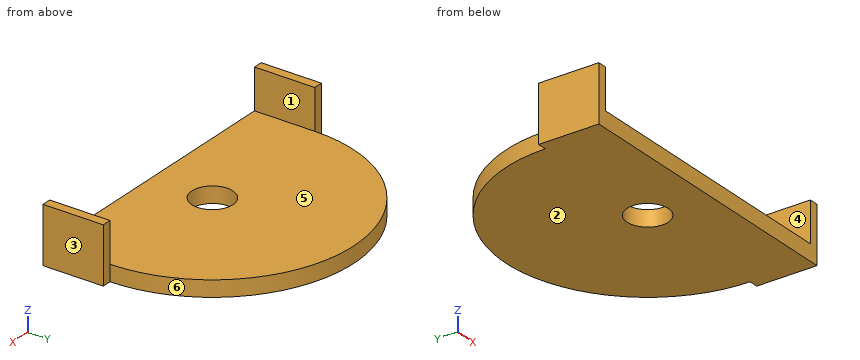
from build123d import *

# Parameters (mm, degrees)
F0_R     = 6.477
F1_DEPTH = 5.08
F2_W     = 2.921
F2_H     = 19.05
F3_DEPTH = 12.7


with BuildPart() as f1:
    # F0 (on Top) → F1 (new body)
    with BuildSketch(Plane.XY):
        with BuildLine():
            Line((47.625, 0), (44.704, 0))
            ThreePointArc((44.704, 0), (0, 44.704), (-44.704, 0))
            Line((-44.704, 0), (-47.625, 0))
            Line((-47.625, 0), (-47.625, -19.05))
            Line((-47.625, -19.05), (47.625, -19.05))
            Line((47.625, -19.05), (47.625, 0))
        make_face()
        Circle(F0_R, mode=Mode.SUBTRACT)
    extrude(amount=F1_DEPTH)

    # F2 (on face) → F3 (join)
    with BuildSketch(Plane.XY.offset(5.08)):
        with Locations((-46.1645, -9.525)):
            Rectangle(F2_W, F2_H)
        with Locations((46.1645, -9.525)):
            Rectangle(F2_W, F2_H)
    extrude(amount=F3_DEPTH)


solid = f1.part
Build history of the part. All positions in model axes, mm. Face numbers are marked on the shaded views. A direction names the side the tool comes from. Round coordinates to 2 decimals unless told otherwise and drop trailing zeros. Write each loop counter-clockwise with the first axis right and the second up, starting at its lowest first coordinate (ties: lowest second). Pieces come first, ordered by that corner, then holes. Notation, with made-up numbers: M 72,75.25 L 89,75.25 A21 ccw 89,83.25 Z; hole C 83.5,56.5 d10. An arc over 180 degrees is marked long. Answer in a Markdown table with one row per item.
1. Saw through at D-D (y = -12). List the corners of the cut face in (x, z) (3 decimals), and give its area (3 significant figures).
Geometry check:
| item | result |
|---|---|
| outline | M -47.625,0 L 47.625,0 L 47.625,17.78 L 44.704,17.78 L 44.704,5.08 L -44.704,5.08 L -44.704,17.78 L -47.625,17.78 Z |
| area | 558 mm2 |
2. Mould opens along X. For the marked faces 1, 2, 3 and 4 say: +X half, -X half, draft (parallel to the pull), parting line (faces both ways), or undercut.
Geometry check:
| item | result |
|---|---|
| face 1 | undercut |
| face 2 | draft |
| face 3 | +X half |
| face 4 | undercut |
3. Which spindle directions (+Z, -Z, +X, -X, +Y, -Y) get a long thin tool onto all of the face, cutting with end or side? Do the marked faces 5 and 6. Say none if no direction does.
Geometry check:
| item | result |
|---|---|
| face 5 | +Z, +Y, -Y |
| face 6 | +Z, -Z, +Y |
4. Flat gauge pins, fed straight in: P1, Ø3, axis at x = 46.5, z = 7.5, coming from the +Y side; P2, Ø4, axis at y = 6, z = 4.5, coming from the -X side; P3, Ø4, axis at x = 14, y = 19, coming from the +Z side; P4, Ø15, axis at x = 0, y = 0, coming from the -Z side. Where does each tip first touch, or does it go through?
Geometry check:
| item | result |
|---|---|
| P1 | y = 0 |
| P2 | x = -44.52 |
| P3 | z = 5.08 |
| P4 | z = 0 |
5. Probe L1, parallel to Y at x = 0, z = 1.9; L2, parallel to Z at x = 43, y = 3; L3, parallel to Y at x = 3, z = 4.5. List the from-to ranges inside material, lowest first. Write a range as [from, to].
Geometry check:
| item | result |
|---|---|
| L1 | [-19.05, -6.48], [6.48, 44.7] |
| L2 | [0, 5.08] |
| L3 | [-19.05, -5.74], [5.74, 44.6] |
6. Saw through at C-C (z = 2.75). List the corners of the cut face in (x, y) (3 decimals), and give its area (3 significant figures).
Geometry check:
| item | result |
|---|---|
| outline | M -47.625,-19.05 L 47.625,-19.05 L 47.625,0 L 44.704,0 A44.704 ccw -44.704,0 L -47.625,0 Z; hole C 0,0 d12.954 |
| area | 4,820 mm2 |
7. Saw through at A-A (x = 0). List the corners of the cut face in (y, z).
Geometry check:
| item | result |
|---|---|
| outline | M -19.05,0 L -6.48,0 L -6.48,5.08 L -19.05,5.08 Z; M 6.48,0 L 44.7,0 L 44.7,5.08 L 6.48,5.08 Z |
8. Saw through at B-B (z = 15). List the corners of the cut face in (x, y) (3 decimals).
Geometry check:
| item | result |
|---|---|
| outline | M -47.625,-19.05 L -44.704,-19.05 L -44.704,0 L -47.625,0 Z; M 44.704,-19.05 L 47.625,-19.05 L 47.625,0 L 44.704,0 Z |
